The listing builds one solid part. Answer for the finished solid, in the listing's coordinates (mm). A direction names the side the tool comes from. Round coordinates to 2 decimals unless told otherwise and drop trailing zeros. Order: outer loops, then holes, each group sorted by start corner. A loop starts at its lowest first (then second) coordinate and runs counter-clockwise, first axis right, second up. Notation, with made-up numbers: (-33, 11) - (-9, 11) arc R3 cw to (-9, 15) - close; hole circle Ø10 at (-22.75, 13). An arc over 180 degrees is marked (long way). One line per item, written item: value. Start each with the question number.
1. A tool of negligible diameter and unlimited length cuts with its end or side. For faces 3 (the flat face through (53, 8.85, 21)), 4 (the flat face through (-51, 9, 33)), from which of +Z, -Z, +X, -X, +Y, -Y can it reach the whole face along a straight path? Write none if from no direction.
2. For a pull along X with two mould halves and no side action, classify faces 1 (the cylindrical face through (10.98, 5.46, 25.03)), 2 (the flat face through (50, 16, -28)) as released by +X, released by -X, zero draft, split by the parting line, or undercut.
3. Straight lines are drawn through the part: line 1 (X direction, y = 11.5, z = 32); line 2 (X direction, y = 13, z = 22); line 3 (Z direction, x = 48, y = 5.45). For each, find the intervals that lie inside material, in ascending order.
4. Section A-A, the plane z = -12.5 is taken. Give the vertices of the cut face in (x, y).
5. Section B-B, the plane x = -13.5 is taken. Give the vertices of the cut face in (y, z), then the cut area to 3 significant figures.
6. Flat-ended cylindrical pins translate along their axes: P1, Ø23, axis at x = 40, z = -9.5, coming from the +Y side; P2, Ø1.5, axis at x = -13, y = 3, coming from the -Z side; P3, Ø1.6, axis at x = 36.5, y = 0.5, coming from the -Z side; P4, Ø2.5, axis at x = -47, z = 32, coming from the +Y side. Find the tip coordinate at first contact, or state that the pin passes through.
7. Section C-C, the plane z = 11.5 is taken. Give the vertices of the cut face in (x, y), then the cut area to 3 significant figures.
from build123d import *

# Parameters (mm, degrees)
SKETCH1_W                   = 120
SKETCH1_H                   = 75
MAIN_STRUCTURE_DEPTH        = 15
SKETCH2_W                   = 116
SKETCH2_H                   = 71
INSIDE_CUT_DEPTH            = 12
SKETCH3_R                   = 2.5
SKETCH3_R_2                 = 1.15
PI_STANDOFFS_DEPTH          = 5
SKETCH4_R                   = 2
SKETCH4_R_2                 = 0.9
CAMERA_STANDOFFS_DEPTH      = 5
BODY_FILLET_1_R             = 4
BODY_FILLET_2_R             = 4
BODY_FILLET_3_R             = 4
BODY_FILLET_4_R             = 4
SKETCH5_R                   = 2.25
SKETCH5_R_2                 = 1.15
FONA_STANDOFFS_DEPTH        = 13
SKETCH6_W                   = 3
SKETCH6_H                   = 3
CORNER_SUPPORT_DEPTH        = 12
SKETCH8_W                   = 22
SKETCH8_H                   = 5
CHARGER_CUTOUT_DEPTH        = 10
SKETCH9_W                   = 8
SKETCH9_H                   = 7
SKETCH9_W_2                 = 7
MOUNTING_STRUCTURE_DEPTH    = 12
MOUNTING_STRUCTURE_FILLET_R = 2
SKETCH10_R                  = 1.3
CASE_MOUNTING_HOLES_DEPTH   = 15
SKETCH13_R                  = 2.9
CASE_SCREW_HEAD_HOLES_DEPTH = 8.85
SKETCH14_R                  = 14.5
SPEAKER_HOLDER_DEPTH        = 1.5
SOUND_CUTOUT_DEPTH          = 1.5
SKETCH25_R                  = 2.5
MICROPHONE_HOLDER_DEPTH     = 1.5
SKETCH26_R                  = 2
MICROPHONE_CUTOUT_DEPTH     = 1.5
SKETCH27_R                  = 4
CAMERA_CUTOUT_DEPTH         = 10


with BuildPart() as part:
    # Sketch1 → Main Structure (new body)
    with BuildSketch(Plane(origin=(0, 0, 0), x_dir=(1, 0, 0), z_dir=(0, 1, 0))):
        Rectangle(SKETCH1_W, SKETCH1_H)
    extrude(amount=MAIN_STRUCTURE_DEPTH)

    # Sketch2 → Inside Cut (cut)
    with BuildSketch(Plane(origin=(0, 15, 0), x_dir=(1, 0, 0), z_dir=(0, 1, 0))):
        Rectangle(SKETCH2_W, SKETCH2_H)
    extrude(amount=-INSIDE_CUT_DEPTH, mode=Mode.SUBTRACT)

    # Sketch3 → Pi Standoffs (add)
    # profile 1 of 4: a face of its own
    with BuildSketch(Plane(origin=(0, 3, 0), x_dir=(1, 0, 0), z_dir=(0, 1, 0))):
        with Locations(Location((-46, -24.5, 0), (0, 0, 90))):
            Circle(SKETCH3_R)
        with Locations(Location((-46, -24.5, 0), (0, 0, 270))):
            Circle(SKETCH3_R_2, mode=Mode.SUBTRACT)
    # profile 2 of 4: a face of its own
    with BuildSketch(Plane(origin=(0, 3, 0), x_dir=(1, 0, 0), z_dir=(0, 1, 0))):
        with Locations(Location((-46, 24.5, 0), (0, 0, 90))):
            Circle(SKETCH3_R)
        with Locations(Location((-46, 24.5, 0), (0, 0, 270))):
            Circle(SKETCH3_R_2, mode=Mode.SUBTRACT)
    # profile 3 of 4: a face of its own
    with BuildSketch(Plane(origin=(0, 3, 0), x_dir=(1, 0, 0), z_dir=(0, 1, 0))):
        with Locations(Location((12, 24.5, 0), (0, 0, 90))):
            Circle(SKETCH3_R)
        with Locations(Location((12, 24.5, 0), (0, 0, 270))):
            Circle(SKETCH3_R_2, mode=Mode.SUBTRACT)
    # profile 4 of 4: a face of its own
    with BuildSketch(Plane(origin=(0, 3, 0), x_dir=(1, 0, 0), z_dir=(0, 1, 0))):
        with Locations(Location((12, -24.5, 0), (0, 0, 90))):
            Circle(SKETCH3_R)
        with Locations(Location((12, -24.5, 0), (0, 0, 270))):
            Circle(SKETCH3_R_2, mode=Mode.SUBTRACT)
    extrude(amount=PI_STANDOFFS_DEPTH)

    # Sketch4 → Camera Standoffs (add)
    # profile 1 of 2: a face of its own
    with BuildSketch(Plane(origin=(0, 3, 0), x_dir=(1, 0, 0), z_dir=(0, 1, 0))):
        with Locations(Location((48, -30.5, 0), (0, 0, 90))):
            Circle(SKETCH4_R)
        with Locations(Location((48, -30.5, 0), (0, 0, 270))):
            Circle(SKETCH4_R_2, mode=Mode.SUBTRACT)
    # profile 2 of 2: a face of its own
    with BuildSketch(Plane(origin=(0, 3, 0), x_dir=(1, 0, 0), z_dir=(0, 1, 0))):
        with Locations(Location((48, -17.5, 0), (0, 0, 90))):
            Circle(SKETCH4_R)
        with Locations(Location((48, -17.5, 0), (0, 0, 270))):
            Circle(SKETCH4_R_2, mode=Mode.SUBTRACT)
    extrude(amount=CAMERA_STANDOFFS_DEPTH)

    # Body Fillet 1
    body_fillet_1_edges = [part.edges().sort_by_distance(p)[0] for p in [
        (-60, 0, 0),
    ]]
    fillet(body_fillet_1_edges, radius=BODY_FILLET_1_R)

    # Body Fillet 2
    body_fillet_2_edges = [part.edges().sort_by_distance(p)[0] for p in [
        (2, 0, -37.5),
        (-58.828427125, 1.171572875, -37.5),
        (-60, 9.5, -37.5),
    ]]
    fillet(body_fillet_2_edges, radius=BODY_FILLET_2_R)

    # Body Fillet 3
    body_fillet_3_edges = [part.edges().sort_by_distance(p)[0] for p in [
        (2, 0, 37.5),
        (-58.828427125, 1.171572875, 37.5),
        (-60, 9.5, 37.5),
    ]]
    fillet(body_fillet_3_edges, radius=BODY_FILLET_3_R)

    # Body Fillet 4
    body_fillet_4_edges = [part.edges().sort_by_distance(p)[0] for p in [
        (60, 9.5, 37.5),
        (60, 9.5, -37.5),
        (60, 1.171572875, -36.328427125),
        (60, 0, 0),
        (60, 1.171572875, 36.328427125),
    ]]
    fillet(body_fillet_4_edges, radius=BODY_FILLET_4_R)

    # Sketch5 → Fona Standoffs (add)
    # profile 1 of 2: a face of its own
    with BuildSketch(Plane(origin=(0, 3, 0), x_dir=(1, 0, 0), z_dir=(0, 1, 0))):
        with Locations(Location((24.33, 29.5, 0), (0, 0, 90))):
            Circle(SKETCH5_R)
        with Locations(Location((24.33, 29.5, 0), (0, 0, 90))):
            Circle(SKETCH5_R_2, mode=Mode.SUBTRACT)
    # profile 2 of 2: a face of its own
    with BuildSketch(Plane(origin=(0, 3, 0), x_dir=(1, 0, 0), z_dir=(0, 1, 0))):
        with Locations(Location((51, 29.5, 0), (0, 0, 90))):
            Circle(SKETCH5_R)
        with Locations(Location((51, 29.5, 0), (0, 0, 90))):
            Circle(SKETCH5_R_2, mode=Mode.SUBTRACT)
    extrude(amount=FONA_STANDOFFS_DEPTH)

    # Sketch6 → Corner Support (add)
    with BuildSketch(Plane(origin=(0, 3, 0), x_dir=(1, 0, 0), z_dir=(0, 1, 0))):
        with Locations((-56.5, -34)):
            Rectangle(SKETCH6_W, SKETCH6_H)
        with Locations((-56.5, 34)):
            Rectangle(SKETCH6_W, SKETCH6_H)
        with Locations((56.5, -34)):
            Rectangle(SKETCH6_W, SKETCH6_H)
        with Locations((56.5, 34)):
            Rectangle(SKETCH6_W, SKETCH6_H)
    extrude(amount=CORNER_SUPPORT_DEPTH)

    # Sketch8 → Charger Cutout (cut)
    with BuildSketch(Plane(origin=(60, 0, 0), x_dir=(0, 0, -1), z_dir=(1, 0, 0))):
        with Locations((4.5, 12.5)):
            Rectangle(SKETCH8_W, SKETCH8_H)
    extrude(amount=-CHARGER_CUTOUT_DEPTH, mode=Mode.SUBTRACT)

    # Sketch9 → Mounting Structure (add)
    with BuildSketch(Plane(origin=(0, 3, 0), x_dir=(1, 0, 0), z_dir=(0, 1, 0))):
        with Locations((-47, -32)):
            Rectangle(SKETCH9_W, SKETCH9_H)
        with Locations((54.5, -22)):
            Rectangle(SKETCH9_W_2, SKETCH9_H)
        with Locations((-47, 32)):
            Rectangle(SKETCH9_W, SKETCH9_H)
        with Locations((14, 32)):
            Rectangle(SKETCH9_W, SKETCH9_H)
        with Locations((14, -32)):
            Rectangle(SKETCH9_W, SKETCH9_H)
    extrude(amount=MOUNTING_STRUCTURE_DEPTH)

    # Mounting Structure Fillet
    mounting_structure_fillet_edges = [part.edges().sort_by_distance(p)[0] for p in [
        (-43, 9, 28.5),
        (-51, 9, 28.5),
        (51, 9, 18.5),
        (51, 9, 25.5),
        (-43, 9, -28.5),
        (-51, 9, -28.5),
        (18, 9, -28.5),
        (10, 9, -28.5),
        (18, 9, 28.5),
        (10, 9, 28.5),
    ]]
    fillet(mounting_structure_fillet_edges, radius=MOUNTING_STRUCTURE_FILLET_R)

    # Sketch10 → Case Mounting Holes (cut)
    with BuildSketch(Plane(origin=(0, 15, 0), x_dir=(1, 0, 0), z_dir=(0, 1, 0))):
        with Locations(Location((-47, 32, 0), (0, 0, 270))):
            Circle(SKETCH10_R)
        with Locations(Location((-47, -32, 0), (0, 0, 270))):
            Circle(SKETCH10_R)
        with Locations(Location((14, -32, 0), (0, 0, 270))):
            Circle(SKETCH10_R)
        with Locations(Location((14, 32, 0), (0, 0, 270))):
            Circle(SKETCH10_R)
        with Locations(Location((54.5, -22, 0), (0, 0, 270))):
            Circle(SKETCH10_R)
    extrude(amount=-CASE_MOUNTING_HOLES_DEPTH, mode=Mode.SUBTRACT)

    # Sketch13 → Case Screw Head Holes (cut)
    with BuildSketch(Plane.XZ):
        with Locations(Location((-47, 32, 0), (0, 0, 270))):
            Circle(SKETCH13_R)
        with Locations(Location((14, 32, 0), (0, 0, 270))):
            Circle(SKETCH13_R)
        with Locations(Location((14, -32, 0), (0, 0, 270))):
            Circle(SKETCH13_R)
        with Locations(Location((-47, -32, 0), (0, 0, 270))):
            Circle(SKETCH13_R)
        with Locations(Location((54.5, 22, 0), (0, 0, 270))):
            Circle(SKETCH13_R)
    extrude(amount=-CASE_SCREW_HEAD_HOLES_DEPTH, mode=Mode.SUBTRACT)

    # Sketch14 → Speaker Holder (cut)
    with BuildSketch(Plane(origin=(0, 3, 0), x_dir=(1, 0, 0), z_dir=(0, 1, 0))):
        with Locations(Location((39, 12.5, 0), (0, 0, 270))):
            Circle(SKETCH14_R)
    extrude(amount=-SPEAKER_HOLDER_DEPTH, mode=Mode.SUBTRACT)

    # Sketch23 → Sound Cutout (cut)
    with BuildSketch(Plane(origin=(0, 1.5, 0), x_dir=(1, 0, 0), z_dir=(0, 1, 0))):
        with BuildLine():
            Line((33, 21), (45, 21))
            ThreePointArc((45, 21), (46.5, 19.5), (45, 18))
            Line((45, 18), (33, 18))
            ThreePointArc((33, 18), (31.5, 19.5), (33, 21))
        make_face()
        with BuildLine():
            Line((30.5, 14), (47.5, 14))
            ThreePointArc((47.5, 14), (49, 12.5), (47.5, 11))
            Line((47.5, 11), (30.5, 11))
            ThreePointArc((30.5, 11), (29, 12.5), (30.5, 14))
        make_face()
        with BuildLine():
            Line((33, 7), (45, 7))
            ThreePointArc((45, 7), (46.5, 5.5), (45, 4))
            Line((45, 4), (33, 4))
            ThreePointArc((33, 4), (31.5, 5.5), (33, 7))
        make_face()
    extrude(amount=-SOUND_CUTOUT_DEPTH, mode=Mode.SUBTRACT)

    # Sketch25 → Microphone holder (cut)
    with BuildSketch(Plane(origin=(0, 3, 0), x_dir=(1, 0, 0), z_dir=(0, 1, 0))):
        with Locations(Location((-51.147743093, 0, 0), (0, 0, 270))):
            Circle(SKETCH25_R)
    extrude(amount=-MICROPHONE_HOLDER_DEPTH, mode=Mode.SUBTRACT)

    # Sketch26 → Microphone Cutout (cut)
    with BuildSketch(Plane(origin=(0, 1.5, 0), x_dir=(1, 0, 0), z_dir=(0, 1, 0))):
        with Locations(Location((-51.147743093, 0, 0), (0, 0, 270))):
            Circle(SKETCH26_R)
    extrude(amount=-MICROPHONE_CUTOUT_DEPTH, mode=Mode.SUBTRACT)

    # Sketch27 → Camera Cutout (cut)
    with BuildSketch(Plane(origin=(0, 3, 0), x_dir=(1, 0, 0), z_dir=(0, 1, 0))):
        with Locations(Location((37.5, -18, 0), (0, 0, 270))):
            Circle(SKETCH27_R)
    extrude(amount=-CAMERA_CUTOUT_DEPTH, mode=Mode.SUBTRACT)


solid = part.part
Answer list:
1. face 3: -Y
1. face 4: +Y
2. face 1: undercut
2. face 2: zero draft
3. line 1: x = -60 to -58, -51 to -48.3, -45.7 to -43, 10 to 12.7, 15.3 to 18, 58 to 60
3. line 2: x = -60 to -58, 51 to 53.2, 55.8 to 60
3. line 3: z = -37.5 to -35.5, 15.5 to 16.6, 18.4 to 19.5, 28.5 to 29.6, 31.4 to 32.5, 35.5 to 37.5
4. outline: (-60, 4) arc R4 ccw to (-56, 0) - (29, 0) - (29, 1.5) - (24.5, 1.5) - (24.5, 3) - (-58, 3) - (-58, 15) - (-60, 15) - close; (49, 0) - (56, 0) arc R4 ccw to (60, 4) - (60, 10) - (58, 10) - (58, 3) - (53.5, 3) - (53.5, 1.5) - (49, 1.5) - close
5. outline: (0, -33.5) arc R4 ccw to (4, -37.5) - (15, -37.5) - (15, -35.5) - (3, -35.5) - (3, 35.5) - (15, 35.5) - (15, 37.5) - (4, 37.5) arc R4 ccw to (0, 33.5) - close
5. area: 266 mm²
6. P1: stops at y = 3
6. P2: stops at z = -37.49
6. P3: stops at z = -36.45
6. P4: passes through
7. outline: (-60, 4) arc R4 ccw to (-56, 0) - (56, 0) arc R4 ccw to (60, 4) - (60, 15) - (58, 15) - (58, 3) - (-58, 3) - (-58, 15) - (-60, 15) - close
7. area: 401 mm²
